from build123d import *

# Parameters (mm, degrees)
SKETCH_1_W            = 52
SKETCH_1_H            = 46
SKETCH_1_R            = 2.6
SKETCH_1_R_2          = 4.15
EXTRUDE_436_DEPTH     = 4
SKETCH_4_R            = 2.1
CUT_EXTRUDE_686_DEPTH = 5
SKETCH_6_R            = 2.1
EXTRUDE_1_DEPTH       = 4
SKETCH_7_R            = 1.2
CUT_EXTRUDE_1_DEPTH   = 5
SKETCH_8_W            = 29.384652785
SKETCH_8_H            = 46
EXTRUDE_2_DEPTH       = 4
SKETCH_9_W            = 29.384652785
SKETCH_9_H            = 46
CUT_EXTRUDE_2_DEPTH   = 5
FILLET_1_R            = 5


with BuildPart() as part:
    # 草图1 → Extrude 436 (new body)
    with BuildSketch(Plane(origin=(0, 0, 0), x_dir=(1, 0, 0), z_dir=(0, 1, 0))):
        Rectangle(SKETCH_1_W, SKETCH_1_H)
        with Locations((-18.25, 0)):
            Circle(SKETCH_1_R, mode=Mode.SUBTRACT)
        with Locations((18.25, 0)):
            Circle(SKETCH_1_R, mode=Mode.SUBTRACT)
        Circle(SKETCH_1_R_2, mode=Mode.SUBTRACT)
    extrude(amount=EXTRUDE_436_DEPTH)

    # 草图4 → Cut-Extrude 686 (cut, through all)
    with BuildSketch(Plane(origin=(0, 4, 0), x_dir=(1, 0, 0), z_dir=(0, 1, 0))):
        with Locations((-12, 18)):
            Circle(SKETCH_4_R)
        with Locations((12, 18)):
            Circle(SKETCH_4_R)
        with Locations((12, -18)):
            Circle(SKETCH_4_R)
        with Locations((-12, -18)):
            Circle(SKETCH_4_R)
    extrude(amount=-CUT_EXTRUDE_686_DEPTH, mode=Mode.SUBTRACT)

    # 草图6 → 凸台-拉伸1 (add)
    with BuildSketch(Plane(origin=(0, 4, 0), x_dir=(1, 0, 0), z_dir=(0, 1, 0))):
        with Locations((-12, -18)):
            Circle(SKETCH_6_R)
        with Locations((12, -18)):
            Circle(SKETCH_6_R)
    extrude(amount=-EXTRUDE_1_DEPTH)

    # 草图7 → 切除-拉伸1 (cut, through all)
    with BuildSketch(Plane(origin=(0, 4, 0), x_dir=(1, 0, 0), z_dir=(0, 1, 0))):
        with Locations((5, -20)):
            Circle(SKETCH_7_R)
        with Locations((-15, -20)):
            Circle(SKETCH_7_R)
    extrude(amount=-CUT_EXTRUDE_1_DEPTH, mode=Mode.SUBTRACT)

    # 草图8 → 凸台-拉伸2 (add)
    with BuildSketch(Plane.XZ):
        with Locations((40.692326393, 0)):
            Rectangle(SKETCH_8_W, SKETCH_8_H)
    extrude(amount=-EXTRUDE_2_DEPTH)

    # 草图9 → 切除-拉伸2 (cut, through all)
    with BuildSketch(Plane(origin=(0, 4, 0), x_dir=(1, 0, 0), z_dir=(0, 1, 0))):
        with Locations((40.692326393, 0)):
            Rectangle(SKETCH_9_W, SKETCH_9_H)
    extrude(amount=-CUT_EXTRUDE_2_DEPTH, mode=Mode.SUBTRACT)

    # 圆角1
    fillet_1_edges = [part.edges().sort_by_distance(p)[0] for p in [
        (-26, 2, 23),
        (-26, 2, -23),
        (26, 2, 23),
        (26, 2, -23),
    ]]
    fillet(fillet_1_edges, radius=FILLET_1_R)


solid = part.part
Input: part model. Units: mm. Frame: model coordinates. Coordinates: 2 decimals unless noted, no trailing zeros. Order: outer loops, then holes, each group sorted by start corner. A loop starts at its lowest first (then second) coordinate and runs counter-clockwise, first axis right, second up. Notation, with made-up numbers: M -3,15 L 14,15 A10 ccw 14,26 Z; hole C 18,63.5 d9. An arc over 180 degrees is marked long. Answer in a Markdown table with one row per item.
(1) Section query B-B, the plane y = 0.9. Output: boundary loops of the cut face in (x, z), plus the area to 3 significant figures.
Numbers:
| item | result |
|---|---|
| outline | M -26,-18 A5 ccw -21,-23 L 21,-23 A5 ccw 26,-18 L 26,18 A5 ccw 21,23 L -21,23 A5 ccw -26,18 Z; hole C -18.25,0 d5.2; hole C -15,20 d2.4; hole C -12,-18 d4.2; hole C 0,0 d8.3; hole C 5,20 d2.4; hole C 12,-18 d4.2; hole C 18.25,0 d5.2 |
| area | 2,240 mm^2 |
(2) Section query C-C, the plane z = 20. Output: boundary loops of the cut face in (x, y).
Numbers:
| item | result |
|---|---|
| outline | M -25.58,0 L -16.2,0 L -16.2,4 L -25.58,4 Z; M -13.8,0 L 3.8,0 L 3.8,4 L -13.8,4 Z; M 6.2,0 L 25.58,0 L 25.58,4 L 6.2,4 Z |
(3) Section query D-D, the plane x = 0. Output: boundary loops of the cut face in (y, z), plus the area to 3 significant figures.
Numbers:
| item | result |
|---|---|
| outline | M 0,-23 L 4,-23 L 4,-4.15 L 0,-4.15 Z; M 0,4.15 L 4,4.15 L 4,23 L 0,23 Z |
| area | 151 mm^2 |
(4) Contact query for a flat-ended pin moving along its axis: pin 1 Ø3.5 at (x, z) = (12, -18) entering from -Y. Output: stop coordinate, or through.
Numbers:
| item | result |
|---|---|
| pin 1 | passes through |
(5) Section query A-A, the plane x = -18.25. Output: boundary loops of the cut face in (y, z), plus the area to 3 significant figures.
Numbers:
| item | result |
|---|---|
| outline | M 0,-23 L 4,-23 L 4,-2.6 L 0,-2.6 Z; M 0,2.6 L 4,2.6 L 4,23 L 0,23 Z |
| area | 163 mm^2 |
(6) Draft query along Z for faces 1 (the flat face through (0, 2, -23)), 2 (the cylindrical face through (-15.77, 1.97, -0.78)), 3 (the cylindrical face through (25, 2, 21)), 4 (the cylindrical face through (4.74, 2.03, 21.17)). Return one class per face: pulls with the +Z half, pulls with the -Z half, needs draft (parallel to the pull), parting line crosses it, or undercut.
Numbers:
| item | result |
|---|---|
| face 1 | pulls with the -Z half |
| face 2 | undercut |
| face 3 | pulls with the +Z half |
| face 4 | undercut |
(7) Material intervals for line 1 (X direction, y = 3.2, z = 0); line 2 (X direction, y = 1.35, z = -18); line 3 (Z direction, x = -12, y = 2), sorted ascending. Write a range as [from, to].
Numbers:
| item | result |
|---|---|
| line 1 | x = [-26, -20.85], [-15.65, -4.15], [4.15, 15.65], [20.85, 26] |
| line 2 | x = [-26, -14.1], [-9.9, 9.9], [14.1, 26] |
| line 3 | z = [-23, -20.1], [-15.9, 23] |
